from build123d import *

# Parameters (mm, degrees)
BOSS_EXTRUDE1_DEPTH      = 8
BOSS_EXTRUDE2_DEPTH      = 7.2
BOSS_EXTRUDE3_START      = 15.2
SKETCH1_3_R              = 6
BOSS_EXTRUDE3_DEPTH      = 8
SKETCH3_W                = 5
SKETCH3_H                = 23.2
BOSS_EXTRUDE4_DEPTH      = 12
CUT_EXTRUDE1_START       = -3
SKETCH4_R                = 6
CUT_EXTRUDE1_DEPTH       = 3
FILLET1_START            = 20.2
FILLET1_DEPTH            = 3.8
FILLET1_START_2          = 8
FILLET1_2_DEPTH          = 7.2
SKETCH7_R                = 6.25
CUT_EXTRUDE4_DEPTH       = 2
FILLET2_R                = 1.5
M4_CLEARANCE_HOLE1_D     = 4.8
CUT_EXTRUDE5_DEPTH       = 42.917610932
CUT_EXTRUDE6_START       = -12
CUT_EXTRUDE6_DEPTH       = 8
CUT_EXTRUDE7_DEPTH       = 8
BOSS_EXTRUDE5_DEPTH      = 10
CUT_EXTRUDE9_DEPTH       = 60.718970453
CUT_EXTRUDE9_DEPTH_BACK  = 60.718970453
SKETCH17_W               = 27.826832925
SKETCH17_H               = 12.4
FILLET3_R                = 5
CUT_EXTRUDE10_REACH      = 60.303
CUT_EXTRUDE11_START      = -8
CUT_EXTRUDE11_DEPTH      = 8
FILLET6_R                = 8
CUT_EXTRUDE12_DEPTH      = 61.936360284
CUT_EXTRUDE12_DEPTH_BACK = 61.936360284


with BuildPart() as part:
    # Sketch1 → Boss-Extrude1 (new body)
    with BuildSketch(Plane.XY):
        with BuildLine():
            ThreePointArc((0, -6), (20.196152423, 5.660254038), (20.196152423, 28.980762114))
            ThreePointArc((20.196152423, 28.980762114), (12, 31.176914536), (9.803847577, 22.980762114))
            ThreePointArc((9.803847577, 22.980762114), (9.803847577, 11.660254038), (0, 6))
            Line((0, 6), (-15, 6))
            Line((-15, 6), (-15, -6))
            Line((-15, -6), (0, -6))
        make_face()
    extrude(amount=BOSS_EXTRUDE1_DEPTH)

    # Sketch2 → Boss-Extrude2 (add)
    with BuildSketch(Plane.XY.offset(8)):
        with BuildLine():
            Line((9.803847577, 22.980762114), (20.196152423, 28.980762114))
            ThreePointArc((20.196152423, 28.980762114), (12, 31.176914536), (9.803847577, 22.980762114))
        make_face()
    extrude(amount=BOSS_EXTRUDE2_DEPTH)

    # Sketch1<3> → Boss-Extrude3 (add)
    with BuildSketch(Plane.XY.offset(BOSS_EXTRUDE3_START)):
        with Locations((15, 25.980762114)):
            Circle(SKETCH1_3_R)
        with BuildLine():
            ThreePointArc((9.803847577, 22.980762114), (9.803847577, 11.660254038), (0, 6))
            ThreePointArc((0, 6), (4.242640687, 4.242640687), (6, 0))
            ThreePointArc((6, 0), (4.242640687, -4.242640687), (0, -6))
            ThreePointArc((0, -6), (20.196152423, 5.660254038), (20.196152423, 28.980762114))
            ThreePointArc((20.196152423, 28.980762114), (20.795554958, 27.533676384), (21, 25.980762114))
            ThreePointArc((21, 25.980762114), (16.552914271, 20.185207156), (9.803847577, 22.980762114))
        make_face()
        Circle(SKETCH1_3_R)
        with BuildLine():
            Line((0, 6), (-15, 6))
            Line((-15, 6), (-15, -6))
            Line((-15, -6), (0, -6))
            ThreePointArc((0, -6), (-6, 0), (0, 6))
        make_face()
    extrude(amount=BOSS_EXTRUDE3_DEPTH)

    # Sketch3 → Boss-Extrude4 (add)
    with BuildSketch(Plane(origin=(0, 6, 0), x_dir=(1, 0, 0), z_dir=(0, 1, 0))):
        with Locations((-17.5, -11.6)):
            Rectangle(SKETCH3_W, SKETCH3_H)
    extrude(amount=-BOSS_EXTRUDE4_DEPTH)

    # Sketch4 → Cut-Extrude1 (cut)
    with BuildSketch(Plane.XY.offset(23.2).offset(CUT_EXTRUDE1_START)):
        with Locations((15, 25.980762114)):
            Circle(SKETCH4_R)
    extrude(amount=CUT_EXTRUDE1_DEPTH, mode=Mode.SUBTRACT)

    # Fillet1: read off the stored shape, not the designer's step
    # Fillet1 outline → Fillet1 (cut)
    with BuildSketch(Plane.XY.offset(FILLET1_START)):
        with BuildLine():
            ThreePointArc((22.78988481, 22.266945911), (21.753590077, 25.724519955), (20.196152423, 28.980762114))
            ThreePointArc((20.196152423, 28.980762114), (20.998549002, 25.848815632), (20.059212052, 22.755181017))
            ThreePointArc((20.059212052, 22.755181017), (21.58802328, 23.425369524), (22.78988481, 22.266945911))
        make_face()
        with BuildLine():
            ThreePointArc((13.184858447, 20.261910731), (11.240000131, 21.305037466), (9.803847577, 22.980762114))
            ThreePointArc((9.803847577, 22.980762114), (10.742643673, 20.891153677), (11.24153696, 18.655330111))
            ThreePointArc((11.24153696, 18.655330111), (11.775316706, 19.988281703), (13.184858447, 20.261910731))
        make_face()
    extrude(amount=FILLET1_DEPTH, mode=Mode.SUBTRACT)

    # Fillet1 2 outline → Fillet1 2 (cut)
    with BuildSketch(Plane.XY.offset(FILLET1_START_2)):
        with BuildLine():
            ThreePointArc((20.196152423, 28.980762114), (19.614014408, 29.816237449), (18.898979486, 30.541240046))
            ThreePointArc((18.898979486, 30.541240046), (19.417907488, 29.263492998), (18.674234614, 28.102082457))
            Line((18.674234614, 28.102082457), (20.196152423, 28.980762114))
        make_face()
        with BuildLine():
            ThreePointArc((11.325765386, 23.85944177), (9.948117916, 23.79610744), (9.101020514, 24.884385796))
            ThreePointArc((9.101020514, 24.884385796), (9.37137372, 23.902646091), (9.803847577, 22.980762114))
            Line((9.803847577, 22.980762114), (11.325765386, 23.85944177))
        make_face()
    extrude(amount=FILLET1_2_DEPTH, mode=Mode.SUBTRACT)

    # Sketch7 → Cut-Extrude4 (cut)
    with BuildSketch(Plane.XY.offset(23.2)):
        Circle(SKETCH7_R)
    extrude(amount=-CUT_EXTRUDE4_DEPTH, mode=Mode.SUBTRACT)

    # Fillet2
    fillet2_edges = [part.edges().sort_by_distance(p)[0] for p in [
        (-1.75, 6, 22.2),
        (1.412020937, 6.08840676, 22.2),
        (-1.75, -6, 22.2),
        (2.028685625, -5.91159324, 22.2),
    ]]
    fillet(fillet2_edges, radius=FILLET2_R)

    # M4 Clearance Hole1 (through all)
    with Locations(Plane.XY.offset(23.2)):
        with Locations((0, 0), (15, 25.980762114)):
            Hole(M4_CLEARANCE_HOLE1_D / 2)

    # Sketch8 → Cut-Extrude5 (cut, symmetric)
    with BuildSketch(Plane(origin=(0, 6, 0), x_dir=(1, 0, 0), z_dir=(0, 1, 0))):
        with BuildLine():
            Line((-16.389921041, 0), (-20, 0))
            Line((-20, 0), (-20, -7.692132935))
            ThreePointArc((-20, -7.692132935), (-19.052602124, -3.443557315), (-16.389921041, 0))
        make_face()
    cut_extrude5 = extrude(amount=CUT_EXTRUDE5_DEPTH, both=True, mode=Mode.SUBTRACT)

    # Mirror1: Cut-Extrude5 across plane
    add(cut_extrude5.mirror(Plane.XY.offset(11.6)), mode=Mode.SUBTRACT)

    # Sketch12 → Cut-Extrude6 (cut)
    with BuildSketch(Plane(origin=(0, 6, 0), x_dir=(1, 0, 0), z_dir=(0, 1, 0)).offset(CUT_EXTRUDE6_START)):
        Polygon((-20, -6.6), (-20, -16.6), (-16, -18.909401077), (-16, -4.290598923), align=None)
    extrude(amount=CUT_EXTRUDE6_DEPTH, mode=Mode.SUBTRACT)

    # Sketch13 → Cut-Extrude7 (cut)
    with BuildSketch(Plane.XZ.offset(6)):
        Polygon((-16, 4.290598923), (-19.936057883, 6.563083001), (-19.986057883, 6.476480461), (-15.9, 4.117393842), (-15.9, 19.082606158), (-19.986057883, 16.723519539), (-19.936057883, 16.636916999), (-16, 18.909401077), align=None)
    extrude(amount=-CUT_EXTRUDE7_DEPTH, mode=Mode.SUBTRACT)

    # Sketch14 → Boss-Extrude5 (add, symmetric)
    with BuildSketch(Plane.XY.offset(11.6)):
        with BuildLine():
            Line((-15, 6), (-15, 13))
            Line((-15, 13), (-50, 13))
            Line((-50, 13), (-50, 9))
            Line((-50, 9), (-25, 9))
            ThreePointArc((-25, 9), (-21.464466094, 7.535533906), (-20, 4))
            Line((-20, 4), (-20, 6))
            Line((-20, 6), (-15, 6))
        make_face()
    extrude(amount=BOSS_EXTRUDE5_DEPTH, both=True)

    # Sketch17 → Cut-Extrude9 (cut, two sides: drawn at the far end of the back side and taken through both)
    with BuildSketch(Plane.XZ.offset(-9).offset(-CUT_EXTRUDE9_DEPTH_BACK)):
        with Locations((-47.413416463, 11.6)):
            Rectangle(SKETCH17_W, SKETCH17_H)
    extrude(amount=CUT_EXTRUDE9_DEPTH + CUT_EXTRUDE9_DEPTH_BACK, mode=Mode.SUBTRACT)

    # Fillet3
    # the kernel refuses this fillet: 5 mm, written as the material it takes off along each edge
    with BuildSketch(Plane(origin=(-50, 25.1346611, 21.6), x_dir=(1, 0, 0), z_dir=(0, -1, 0))) as fillet3_piece_1:
        with BuildLine():
            CenterArc((4.85386444, -5), FILLET3_R, 90, 76.113459637)
            Line((0, -3.8), (-0.097077289, -3.776))
            ThreePointArc((-0.097077289, -3.776), (-0.1, -1.9), (-0.1, 0))
            Line((-0.1, 0), (0, 0.1))
            Line((0, 0.1), (4.85386444, 0.1))
            Line((4.85386444, 0.1), (4.85386444, 0))
        make_face()
    extrude(amount=28.269322199, mode=Mode.SUBTRACT)
    with BuildSketch(Plane(origin=(-50, 25.1346611, 1.6), x_dir=(1, 0, 0), z_dir=(0, -1, 0))) as fillet3_piece_2:
        with BuildLine():
            CenterArc((4.85386444, 5), FILLET3_R, 193.886540363, 76.113459637)
            Line((0, 3.8), (-0.097077289, 3.776))
            ThreePointArc((-0.097077289, 3.776), (-0.1, 1.9), (-0.1, 0))
            Line((-0.1, 0), (0, -0.1))
            Line((0, -0.1), (4.85386444, -0.1))
            Line((4.85386444, -0.1), (4.85386444, 0))
        make_face()
    extrude(amount=28.269322199, mode=Mode.SUBTRACT)

    # Cut-Extrude10: up to this face of the body (flat: up to its plane)
    cut_extrude10_end = Plane(part.part.faces().sort_by_distance((-8.271042779, 6, 18.958105224))[0])
    # Sketch18 → Cut-Extrude10 (cut, up to the picked face)
    with BuildSketch(Plane(origin=(0, 13, 0), x_dir=(1, 0, 0), z_dir=(0, 1, 0)), mode=Mode.PRIVATE) as cut_extrude10_sk1:
        with BuildLine():
            Line((-15, -8.1), (-18.834635496, -8.1))
            ThreePointArc((-18.834635496, -8.1), (-25.079633495, -6.346950766), (-29.5, -1.6))
            Line((-29.5, -1.6), (-15, -1.6))
            Line((-15, -1.6), (-15, -8.1))
        make_face()
    cut_extrude10_tool1 = split(extrude(cut_extrude10_sk1.sketch, amount=-CUT_EXTRUDE10_REACH, mode=Mode.PRIVATE), bisect_by=cut_extrude10_end, keep=Keep.BOTH, mode=Mode.PRIVATE)
    # Sketch18 → Cut-Extrude10 (cut, up to the picked face)
    with BuildSketch(Plane(origin=(0, 13, 0), x_dir=(1, 0, 0), z_dir=(0, 1, 0)), mode=Mode.PRIVATE) as cut_extrude10_sk2:
        with BuildLine():
            Line((-15, -15.1), (-18.834635496, -15.1))
            ThreePointArc((-18.834635496, -15.1), (-25.079633495, -16.853049234), (-29.5, -21.6))
            Line((-29.5, -21.6), (-15, -21.6))
            Line((-15, -21.6), (-15, -15.1))
        make_face()
    cut_extrude10_tool2 = split(extrude(cut_extrude10_sk2.sketch, amount=-CUT_EXTRUDE10_REACH, mode=Mode.PRIVATE), bisect_by=cut_extrude10_end, keep=Keep.BOTH, mode=Mode.PRIVATE)
    add(cut_extrude10_tool1.solids().sort_by(Axis((-20.984013, 13, 4.465435), (0, -1, 0)))[0], mode=Mode.SUBTRACT)
    add(cut_extrude10_tool2.solids().sort_by(Axis((-20.984013, 13, 18.734565), (0, -1, 0)))[0], mode=Mode.SUBTRACT)

    # Sketch19 → Cut-Extrude11 (cut)
    with BuildSketch(Plane.XZ.offset(6).offset(CUT_EXTRUDE11_START)):
        with BuildLine():
            Line((-20.014032682, 6.377161665), (-15.8, 3.944188762))
            Line((-15.8, 3.944188762), (-15.8, 19.255811238))
            Line((-15.8, 19.255811238), (-20.014032682, 16.822838335))
            ThreePointArc((-20.014032682, 16.822838335), (-20.078485255, 16.166756248), (-20.1, 15.507867065))
            Line((-20.1, 15.507867065), (-20.1, 7.692132935))
            ThreePointArc((-20.1, 7.692132935), (-20.078485255, 7.033243752), (-20.014032682, 6.377161665))
        make_face()
        with BuildLine():
            Line((-19.921174748, 6.439020166), (-15.9, 4.117393842))
            Line((-15.9, 4.117393842), (-15.9, 19.082606158))
            Line((-15.9, 19.082606158), (-19.921174748, 16.760979834))
            ThreePointArc((-19.921174748, 16.760979834), (-19.980274232, 16.135661823), (-20, 15.507867065))
            Line((-20, 15.507867065), (-20, 7.692132935))
            ThreePointArc((-20, 7.692132935), (-19.980274232, 7.064338177), (-19.921174748, 6.439020166))
        make_face(mode=Mode.SUBTRACT)
    extrude(amount=CUT_EXTRUDE11_DEPTH, mode=Mode.SUBTRACT)

    # Fillet6
    fillet6_edges = [part.edges().sort_by_distance(p)[0] for p in [
        (-15, 13, 11.6),
    ]]
    fillet(fillet6_edges, radius=FILLET6_R)

    # Sketch20 → Cut-Extrude12 (cut, two sides: drawn at the far end of the back side and taken through both)
    with BuildSketch(Plane(origin=(0, 6, 0), x_dir=(1, 0, 0), z_dir=(0, 1, 0)).offset(-CUT_EXTRUDE12_DEPTH_BACK)):
        with BuildLine():
            Line((-16.389921041, 0), (-23, 0))
            Line((-23, 0), (-23, -7.353876601))
            ThreePointArc((-23, -7.353876601), (-21.519167163, -7.795866352), (-19.993811725, -8.043881717))
            ThreePointArc((-19.993811725, -8.043881717), (-19.125934643, -3.603451376), (-16.389921041, 0))
        make_face()
        with BuildLine():
            Line((-23, -23.2), (-23, -15.846123399))
            ThreePointArc((-23, -15.846123399), (-21.519167163, -15.404133648), (-19.993811725, -15.156118283))
            ThreePointArc((-19.993811725, -15.156118283), (-19.125934643, -19.596548624), (-16.389921041, -23.2))
            Line((-16.389921041, -23.2), (-23, -23.2))
        make_face()
    extrude(amount=CUT_EXTRUDE12_DEPTH + CUT_EXTRUDE12_DEPTH_BACK, mode=Mode.SUBTRACT)


solid = part.part
Model file for the job. Use its own axes, mm. A direction names the side the tool comes from. Give positions to 0.01 mm unless a question says otherwise; leave off trailing zeros. Order: outer loops, then holes, each group sorted by start corner. A loop starts at its lowest first (then second) coordinate and runs counter-clockwise, first axis right, second up. Notation, with made-up numbers: M 3.25,-38.75 L 34.25,-38.75 A22 ccw 34.25,-20.75 Z; hole C -26.5,87 d11. An arc over 180 degrees is marked long. Write item = value, one per line.
Q1. Cut at B-B, the plane y = 0. List the corners of the cut face in (x, z), then the cut area to 3 significant figures.
Derived:
outline = M -19.9,6.31 A10 ccw -16.39,0 L -2.4,0 L -2.4,8 L -15,8 L -15,15.2 L -2.4,15.2 L -2.4,21.2 L -6.25,21.2 L -6.25,23.2 L -16.39,23.2 A10 ccw -19.9,16.89 L -15.8,19.26 L -15.8,3.94 Z; M 2.4,0 L 15.62,0 L 15.62,8 L 2.4,8 Z; M 2.4,15.2 L 15.62,15.2 L 15.62,23.2 L 6.25,23.2 L 6.25,21.2 L 2.4,21.2 Z
area = 443 mm2
Q2. Two-plate mould, pull along Y, no slides. Class faces 1 (the flat face through (-10, 6, 4)), 2 (the flat face through (-15.8, -2, 11)), 3 (the cylindrical face through (-1.29, 2.024, 3.944)), 4 (the cylindrical face through (9.966, 23.788, 11.55)): pulls with the +Y half, pulls with the -Y half, needs draft (parallel to the pull), parting line crosses it, or undercut.
Derived:
face_1 = pulls with the +Y half
face_2 = needs draft
face_3 = undercut
face_4 = pulls with the -Y half
Q3. Tool access for faces 5 (the cylindrical face through (9.886, 11.805, 3.944)), 6 (the cylindrical face through (21.56, 23.43, 21.68)), 7 (the cylindrical face through (6.153, 1.094, 22.214)), 8 (the flat face through (-20, 3, 12)), 9 (the flat face through (-42, 11, 17.8)): list every direction of +Z, -Z, +X, -X, +Y, -Y with a clear straight run to the whole face (end or side of a thin tool).
Derived:
face_5 = +Z, -Z
face_6 = +Z, +Y
face_7 = +Z
face_8 = +Z, -Z, -X, -Y
face_9 = -X, +Y, -Y
Q4. Cut at A-A, the plane x = -40. List the corners of the cut face in (y, z), then the cut area to 3 significant figures.
Derived:
outline = M 9,1.6 L 13,1.6 L 13,5.4 L 9,5.4 Z; M 9,17.8 L 13,17.8 L 13,21.6 L 9,21.6 Z
area = 30.4 mm2
Q5. Drill centre lines: line 1 (Y direction, x = 0, z = 19.35); line 2 (X direction, y = -2.5, z = 5.5); line 3 (Z direction, x = 3, y = 2.5). Where is each one in solid material? Low to high. Write a range as [from, to].
Derived:
line_1 = [-6, -2.4], [2.4, 6]
line_2 = [-19.76, -18.49], [-15.8, 12.29]
line_3 = [0, 8], [15.2, 21.2]
Q6. Flat gauge pins, fed straight in: pin 1 (2.5 mm diameter, centred on x = -14.5, z = 5, fed in from +Y); pin 2 (6 mm diameter, centred on x = -21.5, y = 2.5, fed in from +Z); pin 3 (8 mm diameter, centred on x = -34.5, y = 4.5, fed in from -Z); pin 4 (1.2 mm diameter, centred on x = -44.5, y = 11, fed in from -Z). Where does each tip first touch, or does it go through?
Derived:
pin_1 = 6
pin_2 = 20.78
pin_3 = through
pin_4 = 1.6
Q7. Cut at D-D, the plane z = 9.5. List the corners of the cut face in (x, y).
Derived:
outline = M -33.5,9 L -25,9 A5 cw -20,4 L -20,2 L -15.8,2 L -15.8,-6 L -15,-6 L -15,5 A8 ccw -23,13 L -33.5,13 Z; M 9.1,24.88 A1.5 ccw 11.33,23.86 L 12.92,24.78 A2.4 cw 17.08,27.18 L 18.67,28.1 A1.5 ccw 18.9,30.54 A6 ccw Z
Q8. Cut at C-C, the plane x = 15. List the corners of the cut face in (y, z).
Derived:
outline = M -0.54,0 L 23.58,0 L 23.58,8 L -0.54,8 Z; M -0.54,15.2 L 23.58,15.2 L 23.58,20.2 L 19.98,20.2 L 19.98,23.2 L -0.54,23.2 Z; M 28.38,0 L 31.98,0 L 31.98,20.2 L 28.38,20.2 Z
